```python
from build123d import *

# Parameters (mm, degrees)
SKETCH_1_W          = 37.4
SKETCH_1_H          = 27.4
EXTRUDE_1_DEPTH     = 7
SHELL_1_T           = -1.2
SKETCH_3_W          = 2
SKETCH_3_H          = 9
CUT_EXTRUDE_1_DEPTH = 3.6
SKETCH_4_W          = 2
SKETCH_4_H          = 10
CUT_EXTRUDE_2_DEPTH = 5.2
SKETCH_5_W          = 4
SKETCH_5_H          = 2
CUT_EXTRUDE_3_DEPTH = 2
SKETCH_6_R          = 0.7
EXTRUDE_2_DEPTH     = 5.8
FILLET_1_R          = 3


with BuildPart() as part:
    # 草图1 → 凸台-拉伸1 (new body)
    with BuildSketch(Plane.XY):
        Rectangle(SKETCH_1_W, SKETCH_1_H)
    extrude(amount=EXTRUDE_1_DEPTH)

    # 抽壳1
    shell_1_openings = [part.faces().sort_by_distance(p)[0] for p in [
        (0, 0, 7),
    ]]
    offset(amount=SHELL_1_T, openings=shell_1_openings, kind=Kind.INTERSECTION)

    # 草图3 → 切除-拉伸1 (cut)
    with BuildSketch(Plane.XY.offset(7)):
        with Locations((-18.02869535, 0)):
            Rectangle(SKETCH_3_W, SKETCH_3_H)
    extrude(amount=-CUT_EXTRUDE_1_DEPTH, mode=Mode.SUBTRACT)

    # 草图4 → 切除-拉伸2 (cut)
    with BuildSketch(Plane.XY.offset(7)):
        with Locations((18.188969671, 0)):
            Rectangle(SKETCH_4_W, SKETCH_4_H)
    extrude(amount=-CUT_EXTRUDE_2_DEPTH, mode=Mode.SUBTRACT)

    # 草图5 → 切除-拉伸3 (cut)
    with BuildSketch(Plane.XY.offset(7)):
        with Locations((1.4, -13.132972029)):
            Rectangle(SKETCH_5_W, SKETCH_5_H)
    extrude(amount=-CUT_EXTRUDE_3_DEPTH, mode=Mode.SUBTRACT)

    # 草图6 → 凸台-拉伸2 (add)
    # profile 1 of 4: a face of its own
    with BuildSketch(Plane.XY.offset(1.2)):
        with BuildLine():
            Line((14.5, -7.3), (17.5, -7.3))
            Line((17.5, -7.3), (17.5, -12.5))
            Line((17.5, -12.5), (12.3, -12.5))
            Line((12.3, -12.5), (12.3, -9.5))
            ThreePointArc((12.3, -9.5), (12.944365081, -7.944365081), (14.5, -7.3))
        make_face()
        with Locations((14.5, -9.5)):
            Circle(SKETCH_6_R, mode=Mode.SUBTRACT)
    # profile 2 of 4: a face of its own
    with BuildSketch(Plane.XY.offset(1.2)):
        with BuildLine():
            Line((-12.3, -12.5), (-17.5, -12.5))
            Line((-17.5, -12.5), (-17.5, -7.3))
            Line((-17.5, -7.3), (-14.5, -7.3))
            ThreePointArc((-14.5, -7.3), (-12.944365081, -7.944365081), (-12.3, -9.5))
            Line((-12.3, -9.5), (-12.3, -12.5))
        make_face()
        with Locations((-14.5, -9.5)):
            Circle(SKETCH_6_R, mode=Mode.SUBTRACT)
    # profile 3 of 4: a face of its own
    with BuildSketch(Plane.XY.offset(1.2)):
        with BuildLine():
            Line((-17.5, 12.5), (-17.5, 7.3))
            Line((-17.5, 7.3), (-14.5, 7.3))
            ThreePointArc((-14.5, 7.3), (-12.944365081, 7.944365081), (-12.3, 9.5))
            Line((-12.3, 9.5), (-12.3, 12.5))
            Line((-12.3, 12.5), (-17.5, 12.5))
        make_face()
        with Locations((-14.5, 9.5)):
            Circle(SKETCH_6_R, mode=Mode.SUBTRACT)
    # profile 4 of 4: a face of its own
    with BuildSketch(Plane.XY.offset(1.2)):
        with BuildLine():
            Line((17.5, 12.5), (17.5, 7.3))
            Line((17.5, 7.3), (14.5, 7.3))
            ThreePointArc((14.5, 7.3), (12.944365081, 7.944365081), (12.3, 9.5))
            Line((12.3, 9.5), (12.3, 12.5))
            Line((12.3, 12.5), (17.5, 12.5))
        make_face()
        with Locations((14.5, 9.5)):
            Circle(SKETCH_6_R, mode=Mode.SUBTRACT)
    extrude(amount=EXTRUDE_2_DEPTH)

    # 圆角1
    fillet_1_edges = [part.edges().sort_by_distance(p)[0] for p in [
        (18.7, -13.7, 3.5),
        (-18.7, -13.7, 3.5),
        (-18.7, 13.7, 3.5),
        (18.7, 13.7, 3.5),
    ]]
    fillet(fillet_1_edges, radius=FILLET_1_R)


solid = part.part
```
For this review, take the finished solid that the model builds, in its own axes (mm). A direction names the side the tool comes from. Coordinates: 2 decimals unless noted, no trailing zeros. Order: outer loops, then holes, each group sorted by start corner. A loop starts at its lowest first (then second) coordinate and runs counter-clockwise, first axis right, second up. Notation, with made-up numbers: (8, -35.75) - (13, -35.75) arc R12 cw to (13, -23.75) - close; hole circle Ø4 at (-14.5, 31). An arc over 180 degrees is marked (long way). Answer as a JSON object with one key per item and string values. Group by question number.
1. Clearance check with flat-ended pins moving along their axes: P1, Ø0.9, axis at y = -11.5, z = 4.5, coming from the +X side; P2, Ø1.3, axis at x = 14.5, y = 9.5, coming from the +Z side; P3, Ø1, axis at x = 18.5, z = 4.5, coming from the -Y side. State where each tip first meets the part, or that it passes through.
2. We need section B-B on x = 1. State the section outline as (y, z) points, then the cut area to 3 significant figures.
3. For probe 1 along Y at (x, z) = (14.5, 5); probe 2 along X at (y, z) = (-6, 2); probe 3 along Y at (x, z) = (8.5, 2), list the stretches that pass through material, from the lowest coordinate up.
4. We need section D-D on y = -11.5. State the section outline as (x, z) points.
5. We need section A-A on z = 2.75. Give the number of separate pieces and of enclosed holes in the cut face, then the cut area to 3 significant figures.
6. For faces 4 (the flat face through (0, -12.5, 4)), 5 (the flat face through (18, -5, 4)), 6 (the flat face through (3.4, -13, 6)), 7 (the flat face through (-18, -4.5, 5)), list the 3-axis set-ups (+Z, -Z, +X, -X, +Y, -Y) from which the entire face can be reached by the end or side of a thin tool; tool diameter is ignored.
7. The part is to be moulded in two halves that separate along X. For faces 1 (the flat face through (0, 0, 1.2)), 2 (the flat face through (-18, 4.5, 5)), 3 (the cylindrical face through (17.8, 12.84, 3.55)), say which applies: pulls with the +X half, pulls with the -X half, needs draft (parallel to the pull), parting line crosses it, or undercut.
Final values:
{
 "1": {"P1": "x = 18.68", "P2": "z = 1.2", "P3": "y = -12.63"},
 "2": {"outline": "(-13.7, 0) - (13.7, 0) - (13.7, 7) - (12.5, 7) - (12.5, 1.2) - (-12.5, 1.2) - (-12.5, 5) - (-13.7, 5) - close", "area": "44.4 mm²"},
 "3": {"probe 1": "-13.7 to -10.2, -8.8 to -7.3, 7.3 to 8.8, 10.2 to 13.7", "probe 2": "-18.7 to -17.5, 17.5 to 18.7", "probe 3": "-13.7 to -12.5, 12.5 to 13.7"},
 "4": {"outline": "(-18.59, 0) - (18.59, 0) - (18.59, 7) - (12.3, 7) - (12.3, 1.2) - (-12.3, 1.2) - (-12.3, 7) - (-18.59, 7) - close"},
 "5": {"separate pieces": "1", "enclosed holes": "4", "area": "228 mm²"},
 "6": {"face 4": "+Z", "face 5": "+Z, +X", "face 6": "+Z, -Y", "face 7": "+Z, +X, -X"},
 "7": {"face 1": "undercut", "face 2": "needs draft", "face 3": "pulls with the +X half"}
}
